```python
from build123d import *

# Parameters (mm, degrees)
F2_R     = 3.96875
F3_DEPTH = 25.401
F4_R     = 6.223
F4_R_2   = 3.96875
F5_DEPTH = 8.382


# Not quite as in the source:
# - a feature names something its author has since deleted; it is built from what else it names


with BuildPart() as f1:
    # F0 (on Front) → F1 (revolve)
    with BuildSketch(Plane.XZ):
        Polygon((0, 12.7), (0, 0), (0, -12.7), (9.525, -12.7), (9.525, -2.54), (6.0357036773, -1.27), (6.0357036773, 5.08), (9.525, 6.35), (9.525, 12.7), align=None)
    revolve(axis=Axis((0, 0, 2.3044683039), (0, 0, 1)))

    # F2 (on face) → F3 (cut, through all)
    with BuildSketch(Plane(origin=(0, 0, -12.7), x_dir=(1, 0, 0), z_dir=(0, 0, -1))):
        Circle(F2_R)
    extrude(amount=-F3_DEPTH, mode=Mode.SUBTRACT)

    # F4 (on face) → F5 (cut)
    with BuildSketch(Plane(origin=(0, 0, -12.7), x_dir=(1, 0, 0), z_dir=(0, 0, -1))):
        Circle(F4_R)
        Circle(F4_R_2, mode=Mode.SUBTRACT)
    extrude(amount=-F5_DEPTH, mode=Mode.SUBTRACT)


solid = f1.part
```
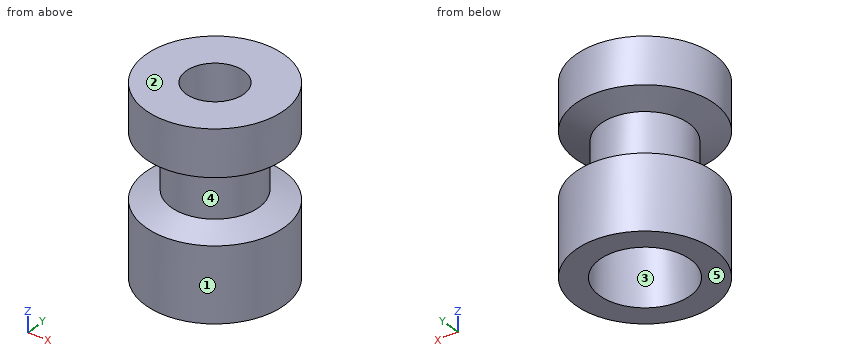
The listing builds one solid part. Answer for the finished solid, in the listing's coordinates (mm). Face numbers are marked on the shaded views. A direction names the side the tool comes from. Give positions to 0.01 mm unless a question says otherwise; leave off trailing zeros. Order: outer loops, then holes, each group sorted by start corner. A loop starts at its lowest first (then second) coordinate and runs counter-clockwise, first axis right, second up. Notation, with made-up numbers: (54.25, 65) -> (112.25, 65) arc R8 cw to (112.25, 70) -> close; hole circle Ø7 at (-27.5, 46.25). An arc over 180 degrees is marked (long way). Answer as a JSON object with one key per item and string values. Group by question number.
Item 1: The part is cut by section A-A on x = 0. Write down the section's boundary in (y, z) (3 decimals), and give its area (3 significant figures).
Item 2: Determine the mould class of the marked faces 1, 2 and 3 for opening direction X: pulls with the +X half, pulls with the -X half, needs draft (parallel to the pull), parting line crosses it, or undercut.
Item 3: Flat-ended cylindrical pins translate along their axes: pin 1 (7.5 mm diameter, centred on x = 0, y = 0, fed in from +Z); pin 2 (6 mm diameter, centred on y = -6, z = -7.5, fed in from -X); pin 3 (2 mm diameter, centred on y = -6, z = -2.5, fed in from +X); pin 4 (1 mm diameter, centred on x = -4, y = 1.5, fed in from -Z). Find the tip coordinate at first contact, or state that the pin passes through.
Item 4: Consider L1, parallel to Y at x = 0, z = 5; L2, parallel to Y at x = 0, z = -7.5 (3 decimals); L3, parallel to X at y = -0.75, z = 0.5. Determine where each line is inside the solid, lowest interval first. Write a range as from..to.
Item 5: A tool of negligible diameter and unlimited length cuts with its end or side. For the marked faces 4 and 5, from which of +Z, -Z, +X, -X, +Y, -Y can it reach the whole face along a straight path? Write none if from no direction.
Item 6: The part is cut by section D-D on z = -8.25. Write down the section's boundary in (x, y) (3 decimals).
Result set:
{
 "1": {"outline": "(-9.525, -12.7) -> (-6.223, -12.7) -> (-6.223, -4.318) -> (-3.969, -4.318) -> (-3.969, 12.7) -> (-9.525, 12.7) -> (-9.525, 6.35) -> (-6.036, 5.08) -> (-6.036, -1.27) -> (-9.525, -2.54) -> close; (3.969, -4.318) -> (6.223, -4.318) -> (6.223, -12.7) -> (9.525, -12.7) -> (9.525, -2.54) -> (6.036, -1.27) -> (6.036, 5.08) -> (9.525, 6.35) -> (9.525, 12.7) -> (3.969, 12.7) -> close", "area": "191 mm²"},
 "2": {"face 1": "parting line crosses it", "face 2": "needs draft", "face 3": "undercut"},
 "3": {"pin 1": "through", "pin 2": "x = -9.04", "pin 3": "x = 8.11", "pin 4": "z = -4.32"},
 "4": {"L1": "-6.04..-3.97, 3.97..6.04", "L2": "-9.525..-6.223, 6.223..9.525", "L3": "-5.99..-3.9, 3.9..5.99"},
 "5": {"face 4": "none", "face 5": "-Z, +X, -X, +Y, -Y"},
 "6": {"outline": "circle Ø19.05 at (0, 0); hole circle Ø12.446 at (0, 0)"}
}
